from build123d import *

# Parameters (mm, degrees)
SKETCH1_W           = 6.35
SKETCH1_H           = 50
SKETCH1_H_2         = 49
SKETCH1_W_2         = 45.825573982
SKETCH1_H_3         = 80
SKETCH1_W_3         = 45.139685757
BOSS_EXTRUDE1_DEPTH = 6.35
FILLET1_R           = 1


with BuildPart() as part:
    # Sketch1 → Boss-Extrude1 (new body)
    with BuildSketch(Plane(origin=(0, 0, 0), x_dir=(1, 0, 0), z_dir=(0, 1, 0))):
        Polygon((157.073624904, 348.621301775), (157.073624902, 288.621301775), (162.073624902, 288.621300264), (162.085917882, 238.621301775), (157.085917882, 238.621301775), (157.085917882, 178.621301775), (162.085917882, 178.621301775), (162.085917882, 128.621301775), (157.085917882, 128.621301775), (157.085917882, 68.621301775), (162.085917882, 68.621301775), (162.085917882, 18.621301775), (157.085917882, 18.621301775), (157.085917882, -41.378698225), (162.085917882, -41.378698225), (162.085917882, -91.378698225), (157.085917882, -91.378698225), (157.085917882, -151.378698225), (162.085917882, -151.378698225), (162.085917882, -201.378698225), (157.085917882, -201.378698225), (157.085917882, -260.378698225), (-137.926375098, -260.378698225), (-137.926375098, -201.378698225), (-142.938668078, -201.378698225), (-142.938668078, -151.378698225), (-137.926375098, -151.378698225), (-137.926375098, -91.378698225), (-142.926375098, -91.378698225), (-142.926375098, -41.378698225), (-137.926375098, -41.378698225), (-137.926375098, 18.621301775), (-142.938668078, 18.621301775), (-142.938668078, 68.621301775), (-137.926375098, 68.621301775), (-137.926375098, 128.621301775), (-142.938668078, 128.621301775), (-142.938668078, 178.621301775), (-137.926375098, 178.621301775), (-137.926375098, 238.621301775), (-142.938668078, 238.621301775), (-142.938668078, 288.621301775), (-137.926375096, 288.621301775), (-137.926375096, 348.621301775), align=None)
        with BuildLine():
            Line((-80.468838102, -30.378698225), (-40.468838102, -30.378698225))
            ThreePointArc((-40.468838102, -30.378698225), (-33.39777029, -33.307630413), (-30.468838102, -40.378698225))
            Line((-30.468838102, -40.378698225), (-30.468838102, -80.378698225))
            ThreePointArc((-30.468838102, -80.378698225), (-33.39777029, -87.449766037), (-40.468838102, -90.378698225))
            Line((-40.468838102, -90.378698225), (-80.468838102, -90.378698225))
            ThreePointArc((-80.468838102, -90.378698225), (-87.539905914, -87.449766037), (-90.468838102, -80.378698225))
            Line((-90.468838102, -80.378698225), (-90.468838102, -40.378698225))
            ThreePointArc((-90.468838102, -40.378698225), (-87.539905914, -33.307630413), (-80.468838102, -30.378698225))
        make_face(mode=Mode.SUBTRACT)
        with BuildLine():
            Line((59.585917882, -30.378698225), (99.585917882, -30.378698225))
            ThreePointArc((99.585917882, -30.378698225), (106.656985694, -33.307630413), (109.585917882, -40.378698225))
            Line((109.585917882, -40.378698225), (109.585917882, -80.378698225))
            ThreePointArc((109.585917882, -80.378698225), (106.656985694, -87.449766037), (99.585917882, -90.378698225))
            Line((99.585917882, -90.378698225), (59.585917882, -90.378698225))
            ThreePointArc((59.585917882, -90.378698225), (52.51485007, -87.449766037), (49.585917882, -80.378698225))
            Line((49.585917882, -80.378698225), (49.585917882, -40.378698225))
            ThreePointArc((49.585917882, -40.378698225), (52.51485007, -33.307630413), (59.585917882, -30.378698225))
        make_face(mode=Mode.SUBTRACT)
        with Locations((131.910917882, -176.378698225)):
            Rectangle(SKETCH1_W, SKETCH1_H, mode=Mode.SUBTRACT)
        with Locations((131.910917882, -65.878698225)):
            Rectangle(SKETCH1_W, SKETCH1_H_2, mode=Mode.SUBTRACT)
        with BuildLine():
            Line((-53.19802656, 248.621301775), (2.80197344, 248.621301775))
            ThreePointArc((2.80197344, 248.621301775), (7.751720908, 246.571049243), (9.80197344, 241.621301775))
            Line((9.80197344, 241.621301775), (9.80197344, 185.621301775))
            ThreePointArc((9.80197344, 185.621301775), (7.751720908, 180.671554307), (2.80197344, 178.621301775))
            Line((2.80197344, 178.621301775), (-53.198026561, 178.621301775))
            ThreePointArc((-53.198026561, 178.621301775), (-58.147774029, 180.671554307), (-60.198026561, 185.621301775))
            Line((-60.198026561, 185.621301775), (-60.19802656, 241.621301775))
            ThreePointArc((-60.19802656, 241.621301775), (-58.147774029, 246.571049243), (-53.19802656, 248.621301775))
        make_face(mode=Mode.SUBTRACT)
        with BuildLine():
            Line((59.085917882, 173.621301775), (115.085917882, 173.621301775))
            ThreePointArc((115.085917882, 173.621301775), (120.03566535, 171.571049243), (122.085917882, 166.621301775))
            Line((122.085917882, 166.621301775), (122.085917882, 110.621301775))
            ThreePointArc((122.085917882, 110.621301775), (120.03566535, 105.671554307), (115.085917882, 103.621301775))
            Line((115.085917882, 103.621301775), (59.085917882, 103.621301775))
            ThreePointArc((59.085917882, 103.621301775), (54.136170414, 105.671554307), (52.085917882, 110.621301775))
            Line((52.085917882, 110.621301775), (52.085917882, 166.621301775))
            ThreePointArc((52.085917882, 166.621301775), (54.136170414, 171.571049243), (59.085917882, 173.621301775))
        make_face(mode=Mode.SUBTRACT)
        with Locations((-70.013588107, 23.936670646)):
            Rectangle(SKETCH1_W_2, SKETCH1_H_3, mode=Mode.SUBTRACT)
        with Locations((94.516075004, 23.936670646)):
            Rectangle(SKETCH1_W_3, SKETCH1_H_3, mode=Mode.SUBTRACT)
    extrude(amount=BOSS_EXTRUDE1_DEPTH)

    # Fillet1
    fillet1_edges = [part.edges().sort_by_distance(p)[0] for p in [
        (162.073624902, 3.175, -288.621300264),
        (162.085917882, 3.175, -238.621301775),
        (162.085917882, 3.175, -178.621301775),
        (162.085917882, 3.175, -128.621301775),
        (162.085917882, 3.175, -68.621301775),
        (162.085917882, 3.175, -18.621301775),
        (162.085917882, 3.175, 41.378698225),
        (162.085917882, 3.175, 91.378698225),
        (162.085917882, 3.175, 151.378698225),
        (162.085917882, 3.175, 201.378698225),
        (-142.938668078, 3.175, 201.378698225),
        (-142.938668078, 3.175, 151.378698225),
        (-142.926375098, 3.175, 91.378698225),
        (-142.926375098, 3.175, 41.378698225),
        (-142.938668078, 3.175, -18.621301775),
        (-142.938668078, 3.175, -68.621301775),
        (-142.938668078, 3.175, -128.621301775),
        (-142.938668078, 3.175, -178.621301775),
        (-142.938668078, 3.175, -238.621301775),
        (-142.938668078, 3.175, -288.621301775),
    ]]
    fillet(fillet1_edges, radius=FILLET1_R)


solid = part.part
Model file for the job. Use its own axes, mm. Give positions to 0.01 mm unless a question says otherwise; leave off trailing zeros. Loops run counter-clockwise (first coordinate to the right, second up) from the corner with the lowest first, then second, coordinate; pieces in that order, holes last. Notation, with made-up numbers: (20.25, 7) -> (40.25, 7) arc R22 ccw to (40.25, 15) -> close; hole circle Ø6 at (69, 24). An arc over 180 degrees is marked (long way). Use a Markdown table: item, result. Add a question column.
(1) Wall check: line 1 along X through (y, z) = (3, -37.5); line 2 along X through (y, z) = (1.5, 57); line 3 along X through (y, z) = (1, -218). Give the ranges that are in metal, low to high.
(2) Slice it at C-C on y = 4.5. Give the number of separate pieces and of enclosed holes in the cut face, and give its area (3 significant figures).
(3) Drop flat-ended pins along their axis: pin 1 Ø3 at (y, z) = (4, 21) entering from -X; pin 2 Ø2 at (x, y) = (159.5, 3.5) entering from +Z; pin 3 Ø2 at (x, y) = (-140, 2) entering from -Z. Give the stop position or say it passes through.
(4) Slice it at B-B on x = -19. List the corners of the cut face in (y, z).
(5) Slice it at A-A on z = -119.5. List the corners of the cut face in (x, y).
Filled sheet:
| question | item | result |
|---|---|---|
| 1 | line 1 | -142.94 to -92.93, -47.1 to 71.95, 117.09 to 162.09 |
| 1 | line 2 | -142.93 to -90.47, -30.47 to 49.59, 109.59 to 128.74, 135.09 to 162.09 |
| 1 | line 3 | -137.93 to -60.2, 9.8 to 157.09 |
| 2 | separate pieces | 1 |
| 2 | enclosed holes | 8 |
| 2 | area | 158,000 mm2 |
| 3 | pin 1 | x = -137.93 |
| 3 | pin 2 | z = 201.38 |
| 3 | pin 3 | z = -288.62 |
| 4 | outline | (0, -348.62) -> (6.35, -348.62) -> (6.35, -248.62) -> (0, -248.62) -> close; (0, -178.62) -> (6.35, -178.62) -> (6.35, 260.38) -> (0, 260.38) -> close |
| 5 | outline | (-137.93, 0) -> (52.09, 0) -> (52.09, 6.35) -> (-137.93, 6.35) -> close; (122.09, 0) -> (157.09, 0) -> (157.09, 6.35) -> (122.09, 6.35) -> close |
